Read the model definition and answer for the solid it produces. Units are mm, in the model's axes. Face numbers are marked on the shaded views. A direction names the side the tool comes from. Give positions to 0.01 mm unless a question says otherwise; leave off trailing zeros. Loops run counter-clockwise (first coordinate to the right, second up) from the corner with the lowest first, then second, coordinate; pieces in that order, holes last. Notation, with made-up numbers: (65, 84) - (74, 84) arc R16 cw to (74, 109) - close; hole circle Ø2 at (18.5, -11). An arc over 180 degrees is marked (long way). Use a Markdown table: item, result. Add a question column.
Item 1: Consider probe 1 along Z at (x, y) = (-974, 581) (3 decimals); probe 2 along X at (y, z) = (625, 10.25); probe 3 along Y at (x, z) = (-976, 23.25). Determine where each line is inside the solid, lowest interval first. Write a range as [from, to].
Item 2: A cutting plane is placed at B-B (y = 614.5). Determine the outline of the cut face in (x, z) (3 decimals), plus the area to 3 significant figures.
Item 3: A cutting plane is placed at D-D (y = 594). Determine the outline of the cut face in (x, z) (3 decimals), plus the area to 3 significant figures.
Item 4: A cutting plane is placed at C-C (z = 5.25). Determine the outline of the cut face in (x, y), plus the area to 3 significant figures.
Item 5: For a pull along Z with two mould halves and no side action, classify the marked faces 1, 2, 3 and 4 as +Z half, -Z half, draft (parallel to the pull), parting line (faces both ways), or undercut.
Item 6: A cutting plane is placed at A-A (x = -949). Determine the outline of the cut face in (y, z) (3 decimals).
Item 7: Which of the six approach directions +Z, -Z, +X, -X, +Y, -Y give full straight-line access (tool end or side, diameter ignored) to the marked faces 5 and 6?
from build123d import *

# Parameters (mm, degrees)
SKETCH1_W           = 50.8
SKETCH1_H           = 67.192198053
SKETCH1_R           = 14.2875
BOSS_EXTRUDE1_DEPTH = 25.4
SKETCH2_W           = 44.45
SKETCH2_H           = 19.05
CUT_EXTRUDE1_DEPTH  = 994.32138208


with BuildPart() as part:
    # Sketch1 → Boss-Extrude1 (new body)
    with BuildSketch(Plane.XY):
        with Locations((-965.320655189, 601.353631034)):
            Rectangle(SKETCH1_W, SKETCH1_H)
        with Locations((-965.375181631, 609.54973006)):
            Circle(SKETCH1_R, mode=Mode.SUBTRACT)
    extrude(amount=BOSS_EXTRUDE1_DEPTH)

    # Sketch2 → Cut-Extrude1 (cut, through all)
    with BuildSketch(Plane(origin=(0, 634.94973006, 0), x_dir=(1, 0, 0), z_dir=(0, 1, 0))):
        with Locations((-965.320655189, -12.7)):
            Rectangle(SKETCH2_W, SKETCH2_H)
    extrude(amount=-CUT_EXTRUDE1_DEPTH, mode=Mode.SUBTRACT)


solid = part.part
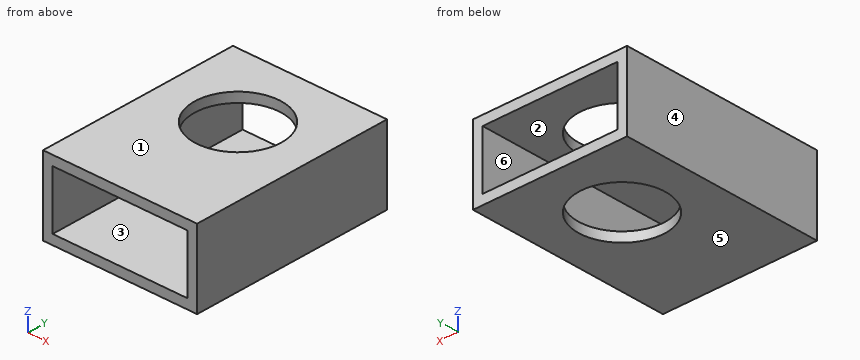
Geometry says:
| question | item | result |
|---|---|---|
| 1 | probe 1 | [0, 3.175], [22.225, 25.4] |
| 1 | probe 2 | [-990.72, -987.55], [-943.1, -939.92] |
| 1 | probe 3 | [567.76, 600], [619.1, 634.95] |
| 2 | outline | (-990.721, 0) - (-978.778, 0) - (-978.778, 3.175) - (-987.546, 3.175) - (-987.546, 22.225) - (-978.778, 22.225) - (-978.778, 25.4) - (-990.721, 25.4) - close; (-951.973, 0) - (-939.921, 0) - (-939.921, 25.4) - (-951.973, 25.4) - (-951.973, 22.225) - (-943.096, 22.225) - (-943.096, 3.175) - (-951.973, 3.175) - close |
| 2 | area | 273 mm² |
| 3 | outline | (-990.721, 0) - (-939.921, 0) - (-939.921, 25.4) - (-990.721, 25.4) - close; hole (-987.546, 3.175) - (-943.096, 3.175) - (-943.096, 22.225) - (-987.546, 22.225) - close |
| 3 | area | 444 mm² |
| 4 | outline | (-990.72, 567.76) - (-987.55, 567.76) - (-987.55, 634.95) - (-990.72, 634.95) - close; (-943.1, 567.76) - (-939.92, 567.76) - (-939.92, 634.95) - (-943.1, 634.95) - close |
| 4 | area | 427 mm² |
| 5 | face 1 | +Z half |
| 5 | face 2 | undercut |
| 5 | face 3 | undercut |
| 5 | face 4 | draft |
| 6 | outline | (567.758, 0) - (634.95, 0) - (634.95, 3.175) - (567.758, 3.175) - close; (567.758, 22.225) - (634.95, 22.225) - (634.95, 25.4) - (567.758, 25.4) - close |
| 7 | face 5 | -Z, +X, -X, +Y, -Y |
| 7 | face 6 | +Y, -Y |
